from build123d import *

# Parameters (mm, degrees)
F0_R     = 27.178
F0_R_2   = 16.002
F1_DEPTH = 25.4
F2_R     = 2.54
F3_R     = 2.54


with BuildPart() as f1:
    # F0 (on Top) → F1 (new body)
    with BuildSketch(Plane.XY):
        Circle(F0_R)
        Circle(F0_R_2, mode=Mode.SUBTRACT)
    extrude(amount=F1_DEPTH)

    # F2
    f2_edges = [f1.edges().sort_by_distance(p)[0] for p in [
        (-27.178, 0, 0),
    ]]
    fillet(f2_edges, radius=F2_R)

    # F3
    f3_edges = [f1.edges().sort_by_distance(p)[0] for p in [
        (-16.002, 0, 0),
        (-27.178, 0, 25.4),
        (-16.002, 0, 25.4),
    ]]
    fillet(f3_edges, radius=F3_R)


solid = f1.part
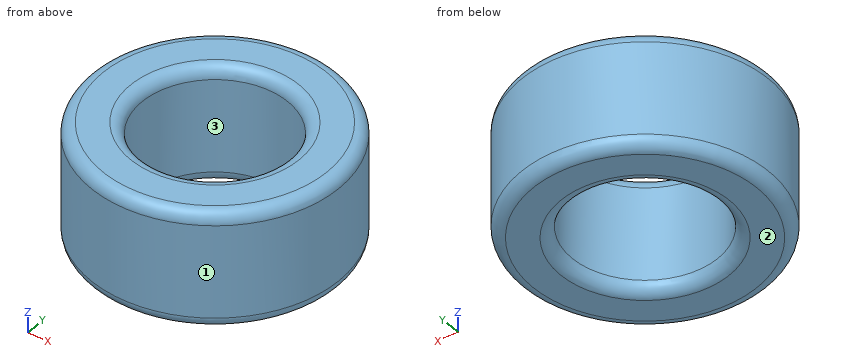
Build history of the part. All positions in model axes, mm. Face numbers are marked on the shaded views. Round coordinates to 2 decimals unless told otherwise and drop trailing zeros. Write each loop counter-clockwise with the first axis right and the second up, starting at its lowest first coordinate (ties: lowest second). Pieces come first, ordered by that corner, then holes. Notation, with made-up numbers: M 57,-2.5 L 74,-2.5 A15 cw 74,6.5 Z; hole C 7.5,11 d9. An arc over 180 degrees is marked long. Answer in a Markdown table with one row per item.
1. Saw through at C-C (z = 14.25). List the corners of the cut face in (x, y), and give its area (3 significant figures).
Geometry check:
| item | result |
|---|---|
| outline | C 0,0 d54.36; hole C 0,0 d32 |
| area | 1,520 mm2 |
2. Probe L1, parallel to Y at x = 0, z = 6.5; L2, parallel to X at y = -5, z = 19.5; L3, parallel to Y at x = -4.5, z = 13.75. List the from-to ranges inside material, lowest first. Write a range as [from, to].
Geometry check:
| item | result |
|---|---|
| L1 | [-27.18, -16], [16, 27.18] |
| L2 | [-26.71, -15.2], [15.2, 26.71] |
| L3 | [-26.8, -15.36], [15.36, 26.8] |
3. Saw through at A-A (y = 0). List the corners of the cut face in (x, z).
Geometry check:
| item | result |
|---|---|
| outline | M -27.18,2.54 A2.54 ccw -24.64,0 L -18.54,0 A2.54 ccw -16,2.54 L -16,22.86 A2.54 ccw -18.54,25.4 L -24.64,25.4 A2.54 ccw -27.18,22.86 Z; M 16,2.54 A2.54 ccw 18.54,0 L 24.64,0 A2.54 ccw 27.18,2.54 L 27.18,22.86 A2.54 ccw 24.64,25.4 L 18.54,25.4 A2.54 ccw 16,22.86 Z |
4. Mould opens along Y. For the marked faces 1, 2 and 3 say: +Y half, -Y half, draft (parallel to the pull), parting line (faces both ways), or undercut.
Geometry check:
| item | result |
|---|---|
| face 1 | parting line |
| face 2 | draft |
| face 3 | undercut |
5. Flat gauge pins, fed straight in: P1, Ø6, axis at x = -5, z = 5, coming from the +Y side; P2, Ø8, axis at y = 10, z = 22.5, coming from the -X side; P3, Ø4, axis at y = -17, z = 10.5, coming from the -X side. Where does each tip first touch, or does it go through?
Geometry check:
| item | result |
|---|---|
| P1 | y = 27.1 |
| P2 | x = -26.51 |
| P3 | x = -22.66 |
